Design review of the part built by this model. Coordinates are the model's own, in mm. A direction names the side the tool comes from. Coordinates: 2 decimals unless noted, no trailing zeros. Loops run counter-clockwise (first coordinate to the right, second up) from the corner with the lowest first, then second, coordinate; pieces in that order, holes last. Notation, with made-up numbers: (81, 74.5) -> (101, 74.5) arc R9 ccw to (101, 84.5) -> close; hole circle Ø1 at (41, 5). An arc over 180 degrees is marked (long way). Use a Markdown table: item, result. Add a question column.
Q1. Take a section at D-D on y = -4.25. Write out the cut boundary in (x, z).
Q2. Clearance check with flat-ended pins moving along their axes: pin 1 Ø4 at (x, y) = (1, 1) entering from +Z; pin 2 Ø2 at (x, y) = (0.5, -4) entering from +Z; pin 3 Ø1.5 at (y, z) = (2, 16) entering from +X; pin 4 Ø2 at (y, z) = (-2, 5.5) entering from -X. State where each tip first meets the part, or that it passes through.
Q3. Draft analysis for pull direction Y (two halves, no side actions). For faces 1 (the face through (-4.86, 1.43, 4.45)), 2 (the face through (5.08, -2.11, 9.86)), 3 (the face through (0, 0, 0)), state which applies: pulls with the +Y half, pulls with the -Y half, needs draft (parallel to the pull), parting line crosses it, or undercut.
Q4. For probe 1 along X at (y, z) = (0, 10); probe 2 along Z at (x, y) = (-4, -1), list the stretches that pass through material, from the lowest coordinate up.
Q5. For faces 4 (the face through (-5, 0, 20)), 5 (the face through (0, 0, 1)), list the 3-axis set-ups (+Z, -Z, +X, -X, +Y, -Y) from which the entire face can be reached by the end or side of a thin tool; tool diameter is ignored.
Q6. Take a section at B-B on x = 0. Write out the cut boundary in (y, z).
Q7. Take a section at C-C on z = 9.5. Write out the cut boundary in (x, y).
Q8. Take a section at A-A on y = 0. Write out the cut boundary in (x, z), plus the area to 3 significant figures.
from build123d import *

# Parameters (mm, degrees)
F0_R     = 5.5
F1_DEPTH = 20
F2_R     = 4.5
F3_DEPTH = 19
F4_R     = 1.5
F5_DEPTH = 25


with BuildPart() as f1:
    # F0 (on Top) → F1 (new body)
    with BuildSketch(Plane.XY):
        Circle(F0_R)
    extrude(amount=F1_DEPTH)

    # F2 (on face) → F3 (cut)
    with BuildSketch(Plane.XY.offset(20)):
        Circle(F2_R)
    extrude(amount=-F3_DEPTH, mode=Mode.SUBTRACT)

    # F4 (on Right) → F5 (cut)
    with BuildSketch(Plane.YZ):
        with Locations((0, 4)):
            Circle(F4_R)
    extrude(amount=-F5_DEPTH, mode=Mode.SUBTRACT)


solid = f1.part
Answer list:
| question | item | result |
|---|---|---|
| 1 | outline | (-3.49, 0) -> (3.49, 0) -> (3.49, 20) -> (1.48, 20) -> (1.48, 1) -> (-1.48, 1) -> (-1.48, 20) -> (-3.49, 20) -> close |
| 2 | pin 1 | z = 1 |
| 2 | pin 2 | z = 20 |
| 2 | pin 3 | x = 5.36 |
| 2 | pin 4 | x = -5.41 |
| 3 | face 1 | undercut |
| 3 | face 2 | parting line crosses it |
| 3 | face 3 | needs draft |
| 4 | probe 1 | -5.5 to -4.5, 4.5 to 5.5 |
| 4 | probe 2 | 0 to 1 |
| 5 | face 4 | +Z, +X, -X, +Y, -Y |
| 5 | face 5 | +Z |
| 6 | outline | (-5.5, 0) -> (5.5, 0) -> (5.5, 20) -> (4.5, 20) -> (4.5, 1) -> (-4.5, 1) -> (-4.5, 20) -> (-5.5, 20) -> close |
| 7 | outline | circle Ø11 at (0, 0); hole circle Ø9 at (0, 0) |
| 8 | outline | (-5.5, 0) -> (5.5, 0) -> (5.5, 20) -> (4.5, 20) -> (4.5, 1) -> (-4.5, 1) -> (-4.5, 2.5) -> (-5.5, 2.5) -> close; (-5.5, 5.5) -> (-4.5, 5.5) -> (-4.5, 20) -> (-5.5, 20) -> close |
| 8 | area | 46.0 mm² |
